Read the model definition and answer for the solid it produces. Units are mm, in the model's axes. Coordinates: 2 decimals unless noted, no trailing zeros. Order: outer loops, then holes, each group sorted by start corner. A loop starts at its lowest first (then second) coordinate and runs counter-clockwise, first axis right, second up. Notation, with made-up numbers: (-10.5, 2.25) -> (-1.5, 2.25) arc R21 ccw to (-1.5, 22.25) -> close; hole circle Ø6 at (86.5, 28). An arc over 180 degrees is marked (long way). Use CSV: the item, a comma, the result in double quotes.
```python
from build123d import *

# Parameters (mm, degrees)
SKETCH1_W           = 165
SKETCH1_H           = 50
BOSS_EXTRUDE1_DEPTH = 2.5
FILLET1_R           = 25
SKETCH2_R           = 2.5
CUT_EXTRUDE1_DEPTH  = 2.5
SKETCH4_R           = 2.25
CUT_EXTRUDE2_DEPTH  = 10


with BuildPart() as part:
    # Sketch1 → Boss-Extrude1 (new body)
    with BuildSketch(Plane.XY):
        Rectangle(SKETCH1_W, SKETCH1_H)
    extrude(amount=BOSS_EXTRUDE1_DEPTH)

    # Fillet1
    fillet1_edges = [part.edges().sort_by_distance(p)[0] for p in [
        (-82.5, -25, 1.25),
        (-82.5, 25, 1.25),
        (82.5, -25, 1.25),
        (82.5, 25, 1.25),
    ]]
    fillet(fillet1_edges, radius=FILLET1_R - 0.0001)  # a hair under: the kernel refuses the full size

    # Sketch2 → Cut-Extrude1 (cut)
    with BuildSketch(Plane.XY.offset(2.5)):
        with Locations((-5, 20)):
            Circle(SKETCH2_R)
        with Locations((5, 20)):
            Circle(SKETCH2_R)
    cut_extrude1 = extrude(amount=-CUT_EXTRUDE1_DEPTH, mode=Mode.SUBTRACT)

    # Mirror1: Cut-Extrude1 across plane
    add(cut_extrude1.mirror(Plane.ZX), mode=Mode.SUBTRACT)

    # Sketch4 → Cut-Extrude2 (cut)
    with BuildSketch(Plane.XY.offset(2.5)):
        with Locations((-57.5, 0)):
            Circle(SKETCH4_R)
    cut_extrude2 = extrude(amount=-CUT_EXTRUDE2_DEPTH, mode=Mode.SUBTRACT)

    # Mirror2: Cut-Extrude2 across plane
    add(cut_extrude2.mirror(Plane(origin=(0, 0, 0), x_dir=(0, 0, 1), z_dir=(1, 0, 0))), mode=Mode.SUBTRACT)


solid = part.part
```
Item 1: Find section C-C, the plane z = 0.7. Give the number of separate pieces and of enclosed holes in the cut face, then the cut area to 3 significant figures.
Return value:
separate pieces,"1"
enclosed holes,"6"
area,"7,600 mm^2"
Item 2: Find section D-D, the plane y = -9. Give the vertices of the cut face in (x, z).
Return value:
outline,"(-80.82, 0) -> (80.82, 0) -> (80.82, 2.5) -> (-80.82, 2.5) -> close"
Item 3: Straight lines are drawn through the part: line 1 along Y through (x, z) = (5, 1.6); line 2 along Y through (x, z) = (-57.5, 0.65); line 3 along X through (y, z) = (20.5, 0.25). For each, find the intervals that lie inside material, in ascending order.
Return value:
line 1,"y = -25 to -22.5, -17.5 to 17.5, 22.5 to 25"
line 2,"y = -25 to -2.25, 2.25 to 25"
line 3,"x = -71.81 to -7.45, -2.55 to 2.55, 7.45 to 71.81"
Item 4: Find section A-A, the plane x = 5. Give the vertices of the cut face in (y, z), then the cut area to 3 significant figures.
Return value:
outline,"(-25, 0) -> (-22.5, 0) -> (-22.5, 2.5) -> (-25, 2.5) -> close; (-17.5, 0) -> (17.5, 0) -> (17.5, 2.5) -> (-17.5, 2.5) -> close; (22.5, 0) -> (25, 0) -> (25, 2.5) -> (22.5, 2.5) -> close"
area,"100 mm^2"
Item 5: Find section B-B, the plane y = 20. Give the vertices of the cut face in (x, z), then the cut area to 4 significant figures.
Return value:
outline,"(-72.5, 0) -> (-7.5, 0) -> (-7.5, 2.5) -> (-72.5, 2.5) -> close; (-2.5, 0) -> (2.5, 0) -> (2.5, 2.5) -> (-2.5, 2.5) -> close; (7.5, 0) -> (72.5, 0) -> (72.5, 2.5) -> (7.5, 2.5) -> close"
area,"337.5 mm^2"
Item 6: The mould has two halves that part along X. Classify faces 1 (the cylindrical face through (74.982, -17.871, 1.268)), 2 (the cylindrical face through (-75.371, -17.482, 1.268)), 3 (the flat face through (-1, 0, 0)), 4 (the cylindrical face through (-3.66, 22.11, 1.27)): +X half, -X half, draft (parallel to the pull), parting line (faces both ways), or undercut.
Return value:
face 1,"+X half"
face 2,"-X half"
face 3,"draft"
face 4,"undercut"
Item 7: This flat-tipped pin is pushed along its axis until it touches: P1, Ø3, axis at x = 5, y = -20, coming from the +Z side. Where does it stop, or does it pass through?
Return value:
P1,"passes through"
